Work out the finished part from the listing and answer in its coordinate system (mm). Face numbers are marked on the shaded views. A direction names the side the tool comes from. Give positions to 0.01 mm unless a question says otherwise; leave off trailing zeros. Order: outer loops, then holes, each group sorted by start corner. A loop starts at its lowest first (then second) coordinate and runs counter-clockwise, first axis right, second up. Notation, with made-up numbers: (52, 33.25) - (102, 33.25) arc R29 ccw to (102, 71.25) - close; hole circle Ø9 at (-8, 52). An arc over 180 degrees is marked (long way). Put each result on its own line as item: value.
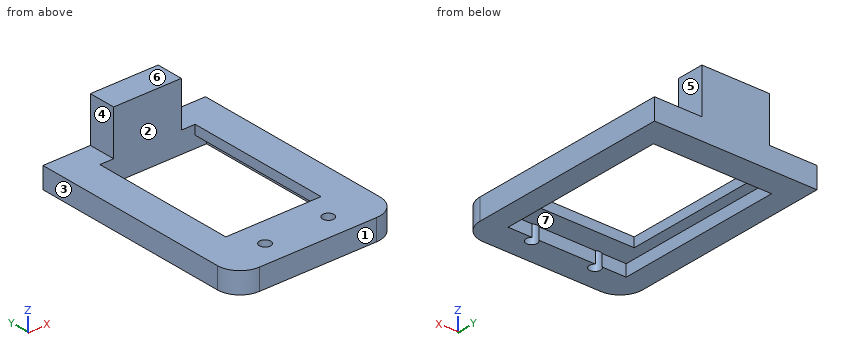
```python
from build123d import *

# Parameters (mm, degrees)
F0_W     = 72
F0_H     = 100
F1_DEPTH = 9.4
F2_W     = 42.2
F2_H     = 65
F3_DEPTH = 5.2
F4_DEPTH = 9.4
F5_W     = 30
F5_H     = 12
F6_DEPTH = 20
F7_R     = 2.5
F8_DEPTH = 9.4
F9_R     = 10


# Not quite as in the source:
# - a feature names something its author has since deleted; it is built from what else it names


with BuildPart() as f1:
    # F0 (on Top) → F1 (new body)
    with BuildSketch(Plane.XY):
        Rectangle(F0_W, F0_H)
    extrude(amount=F1_DEPTH)

    # F2 (on face) → F3 (cut)
    with BuildSketch(Plane(origin=(0, 0, 0), x_dir=(1, 0, 0), z_dir=(0, 0, -1))):
        Polygon((21.1, -38), (26.15, -38), (26.15, 37), (-26.15, 37), (-26.15, -38), (-21.1, -38), (-21.1, 27), (21.1, 27), align=None)
        with Locations((0, -5.5)):
            Rectangle(F2_W, F2_H)
    extrude(amount=-F3_DEPTH, mode=Mode.SUBTRACT)

    # F2 (on face) → F4 (cut, through all)
    with BuildSketch(Plane(origin=(0, 0, 0), x_dir=(1, 0, 0), z_dir=(0, 0, -1))):
        with Locations((0, -5.5)):
            Rectangle(F2_W, F2_H)
    extrude(amount=-F4_DEPTH, mode=Mode.SUBTRACT)

    # F5 (on face) → F6 (join)
    with BuildSketch(Plane.XY.offset(9.4)):
        with Locations((0, 44)):
            Rectangle(F5_W, F5_H)
    extrude(amount=F6_DEPTH)

    # F7 (on face) → F8 (cut, through all)
    with BuildSketch(Plane.XY.offset(9.4)):
        with Locations((-14, -39)):
            Circle(F7_R)
        with Locations((14, -39)):
            Circle(F7_R)
    extrude(amount=-F8_DEPTH, mode=Mode.SUBTRACT)

    # F9
    f9_edges = [f1.edges().sort_by_distance(p)[0] for p in [
        (36, -50, 4.7),
        (-36, -50, 4.7),
    ]]
    fillet(f9_edges, radius=F9_R)


solid = f1.part
```
(1) A tool of negligible diameter and unlimited length cuts with its end or side. For the marked faces 4, 5, 6 and 7, from which of +Z, -Z, +X, -X, +Y, -Y can it reach the whole face along a straight path? Write none if from no direction.
Geometry check:
face 4: +Z, -X, +Y, -Y
face 5: +Z, +X, +Y, -Y
face 6: +Z, +X, -X, +Y, -Y
face 7: -Z
(2) Straight lines are drawn through the part: line 1 (X direction, y = -39, z = 5.5); line 2 (Y direction, x = 14, z = 6); line 3 (Y direction, x = 14, z = 3.5). For each, find the intervals that lie inside material, in ascending order.
Geometry check:
line 1: x = -36 to -16.5, -11.5 to 11.5, 16.5 to 36
line 2: y = -50 to -41.5, -36.5 to -27, 38 to 50
line 3: y = -50 to -41.5, 38 to 50
(3) Given pin 1 (1 mm diameter, centred on x = -23, y = 10, fed in from -Z); pin 2 (15.5 mm diameter, centred on x = 7, y = -14, fed in from -Z); pin 3 (4 mm diameter, centred on x = -24.5, y = -4.5, fed in from +Z); pin 4 (3 mm diameter, centred on x = -2, z = 25.5, fed in from -Y), each flat-ended and moving along its own axis, determine where each tip first touches the part or whether it passes through.
Geometry check:
pin 1: stops at z = 5.2
pin 2: passes through
pin 3: stops at z = 9.4
pin 4: stops at y = 38
(4) Section B-B, the plane y = -14.5 is taken. Write down the section's boundary in (x, z), then the cut area to 3 significant figures.
Geometry check:
outline: (-36, 0) - (-26.15, 0) - (-26.15, 5.2) - (-21.1, 5.2) - (-21.1, 9.4) - (-36, 9.4) - close; (21.1, 5.2) - (26.15, 5.2) - (26.15, 0) - (36, 0) - (36, 9.4) - (21.1, 9.4) - close
area: 228 mm²
(5) Section C-C, the plane z = 20.5 is taken. Write down the section's boundary in (x, y), then the cut area to 3 significant figures.
Geometry check:
outline: (-15, 38) - (15, 38) - (15, 50) - (-15, 50) - close
area: 360 mm²
(6) Determine the mould class of the marked faces 1, 2 and 3 for opening direction X: pulls with the +X half, pulls with the -X half, needs draft (parallel to the pull), parting line crosses it, or undercut.
Geometry check:
face 1: needs draft
face 2: undercut
face 3: pulls with the -X half
(7) Section A-A, the plane x = 2 is taken. Write down the section's boundary in (y, z), then the cut area to 3 significant figures.
Geometry check:
outline: (-50, 0) - (-37, 0) - (-37, 5.2) - (-27, 5.2) - (-27, 9.4) - (-50, 9.4) - close; (38, 0) - (50, 0) - (50, 29.4) - (38, 29.4) - close
area: 517 mm²
